```python
from build123d import *

# Parameters (mm, degrees)
BOSS_EXTRUDE1_DEPTH      = 5
BOSS_EXTRUDE1_DEPTH_BACK = 10
SKETCH1_R                = 35
M3_CLEARANCE_HOLE1_D     = 3.4
CIRPATTERN1_COUNT        = 6
SKETCH4_R                = 30
CUT_EXTRUDE1_DEPTH       = 2
M3_CLEARANCE_HOLE2_D     = 3.4
SKETCH8_R                = 35
SKETCH8_R_2              = 27.5
CUT_EXTRUDE4_DEPTH       = 4
FILLET1_R                = 0.2
SKETCH9_R                = 11.1
CUT_EXTRUDE5_DEPTH       = 10
SKETCH10_R               = 35
SKETCH10_R_2             = 27.5
CUT_EXTRUDE6_DEPTH       = 10
SKETCH11_R               = 26.5
CUT_EXTRUDE7_DEPTH       = 9
SKETCH12_R               = 11.1
CUT_EXTRUDE8_DEPTH       = 9
CHAMFER1_SIZE            = 0.2
CHAMFER2_SIZE            = 3


with BuildPart() as part:
    # Sketch1 → Boss-Extrude1 (new, two sides: drawn at the far end of the back side and taken through both)
    with BuildSketch(Plane.XY.offset(-BOSS_EXTRUDE1_DEPTH_BACK)):
        Circle(SKETCH1_R)
    extrude(amount=BOSS_EXTRUDE1_DEPTH + BOSS_EXTRUDE1_DEPTH_BACK)

    # M3 Clearance Hole1 (through all)
    with Locations(Plane.XY.offset(5)):
        with Locations((0, 32.5)):
            m3_clearance_hole1 = Hole(M3_CLEARANCE_HOLE1_D / 2)

    # CirPattern1: M3 Clearance Hole1 ×6 about axis
    cirpattern1_axis = Axis((0, -0.076854784, 0), (0, 0, 1))
    for i in range(1, CIRPATTERN1_COUNT):
        add(m3_clearance_hole1.rotate(cirpattern1_axis, i * 360 / CIRPATTERN1_COUNT), mode=Mode.SUBTRACT)

    # Sketch4 → Cut-Extrude1 (cut)
    with BuildSketch(Plane.XY.offset(5)):
        Circle(SKETCH4_R)
    extrude(amount=-CUT_EXTRUDE1_DEPTH, mode=Mode.SUBTRACT)

    # M3 Clearance Hole2 (through all)
    with Locations(Plane(origin=(-15.55, 15.55, 3), x_dir=(1, 0, 0), z_dir=(0, 0, 1))):
        with Locations((0, 0), (31.1, 0), (31.1, -31.1), (0, -31.1)):
            Hole(M3_CLEARANCE_HOLE2_D / 2)

    # Sketch8 → Cut-Extrude4 (cut)
    with BuildSketch(Plane(origin=(0, 0, -10), x_dir=(-1, 0, 0), z_dir=(0, 0, -1))):
        with Locations(Location((0, 0, 0), (0, 0, 180))):
            Circle(SKETCH8_R)
        Circle(SKETCH8_R_2, mode=Mode.SUBTRACT)
    extrude(amount=-CUT_EXTRUDE4_DEPTH, mode=Mode.SUBTRACT)

    # Fillet1
    fillet1_edges = [part.edges().sort_by_distance(p)[0] for p in [
        (-35, 0, -6),
        (27.5, 0, -10),
    ]]
    fillet(fillet1_edges, radius=FILLET1_R)

    # Sketch9 → Cut-Extrude5 (cut)
    with BuildSketch(Plane.XY.offset(3)):
        Circle(SKETCH9_R)
    extrude(amount=-CUT_EXTRUDE5_DEPTH, mode=Mode.SUBTRACT)

    # Sketch10 → Cut-Extrude6 (cut)
    with BuildSketch(Plane(origin=(0, 0, -10), x_dir=(-1, 0, 0), z_dir=(0, 0, -1))):
        with Locations(Location((0, 0, 0), (0, 0, 180))):
            Circle(SKETCH10_R)
        Circle(SKETCH10_R_2, mode=Mode.SUBTRACT)
    extrude(amount=-CUT_EXTRUDE6_DEPTH, mode=Mode.SUBTRACT)

    # Sketch11 → Cut-Extrude7 (cut)
    with BuildSketch(Plane.XY.offset(3)):
        Circle(SKETCH11_R)
    extrude(amount=-CUT_EXTRUDE7_DEPTH, mode=Mode.SUBTRACT)

    # Sketch12 → Cut-Extrude8 (cut)
    with BuildSketch(Plane.XY.offset(-7)):
        Circle(SKETCH12_R)
    extrude(amount=-CUT_EXTRUDE8_DEPTH, mode=Mode.SUBTRACT)

    # Chamfer1
    chamfer1_edges = [part.edges().sort_by_distance(p)[0] for p in [
        (-35, 0, 0),
        (-11.1, 0, -6),
    ]]
    chamfer(chamfer1_edges, length=CHAMFER1_SIZE)

    # Chamfer2
    chamfer2_edges = [part.edges().sort_by_distance(p)[0] for p in [
        (-26.5, 0, 3),
    ]]
    chamfer(chamfer2_edges, length=CHAMFER2_SIZE)


solid = part.part
```
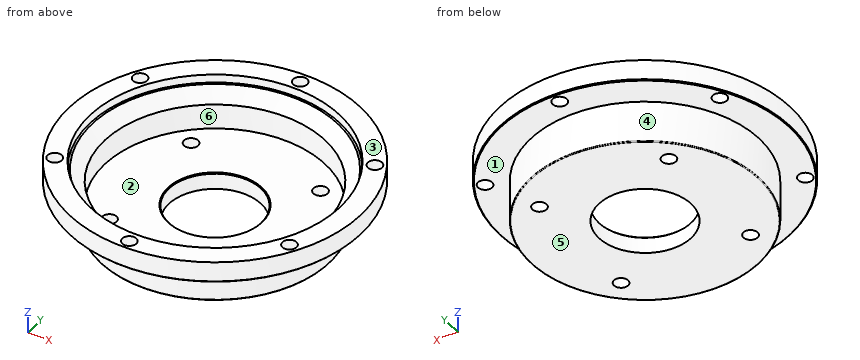
Model file for the job. Use its own axes, mm. Face numbers are marked on the shaded views. A direction names the side the tool comes from. Give positions to 0.01 mm unless a question says otherwise; leave off trailing zeros. Write each loop counter-clockwise with the first axis right and the second up, starting at its lowest first coordinate (ties: lowest second). Pieces come first, ordered by that corner, then holes. Notation, with made-up numbers: (-21, 46) - (2, 46) arc R16 cw to (2, 64) - close; hole circle Ø4 at (-18.5, -27.75). An arc over 180 degrees is marked (long way). One line per question, with ' | ' between items. Start each with the question number.
(1) Pin check, flat tips, straight feed: P1, Ø4.5, axis at x = -28.21, y = -16.37, coming from the +Z side; P2, Ø10, axis at x = 26.5, y = -21, coming from the -Z side; P3, Ø4, axis at x = -2, y = -16, coming from the +Z side; P4, Ø2, axis at x = -3, z = -2.5, coming from the +Y side. Stop position of each tip, or through.
(2) 3-axis set-ups, long thin cutter, end or side, ignore diameter. For the marked faces 1, 2 and 3: which of +Z, -Z, +X, -X, +Y, -Y reach the whole face in a straight line?
(3) Slice it at B-B on z = -8.25. Write the cut outline in (x, y), plus the area to 3 significant figures.
(4) Two-plate mould, pull along X, no slides. Class the marked faces 4, 5 and 6: +X half, -X half, draft (parallel to the pull), parting line (faces both ways), or undercut.
(5) Wall check: line 1 along Y through (x, z) = (0, 3.4); line 2 along Y through (x, z) = (0, -7.65); line 3 along Y through (x, z) = (28, 1). Give the ranges that are in metal, low to high. Write a range as from..to.
(6) Slice it at C-C on x = 15. Give the number of separate pieces and of enclosed holes in the cut face, plus the area to 3 significant figures.
(7) Slice it at A-A on y = 0. Write the cut outline in (x, z).
Results below:
1) P1: z = 5 | P2: z = 0 | P3: z = -6 | P4: y = 27.43
2) face 1: -Z | face 2: +Z | face 3: +Z, +X, -X, +Y, -Y
3) outline: circle Ø55 at (0, 0); hole circle Ø3.4 at (-15.55, -15.55); hole circle Ø3.4 at (-15.55, 15.55); hole circle Ø22.2 at (0, 0); hole circle Ø3.4 at (15.55, -15.55); hole circle Ø3.4 at (15.55, 15.55) | area: 1,950 mm^2
4) face 4: parting line | face 5: draft | face 6: undercut
5) line 1: -35..-34.35, -30.95..-30, 30..30.8, 34.2..35 | line 2: -27.5..-11.1, 11.1..27.5 | line 3: -21..-18.05, -14.68..14.52, 17.9..21
6) separate pieces: 3 | enclosed holes: 0 | area: 244 mm^2
7) outline: (-35, 0.2) - (-34.8, 0) - (-27.5, 0) - (-27.5, -9.8) arc R0.2 ccw to (-27.3, -10) - (-11.1, -10) - (-11.1, -6.2) - (-11.3, -6) - (-26.5, -6) - (-26.5, 0) - (-29.5, 3) - (-30, 3) - (-30, 5) - (-35, 5) - close; (11.1, -10) - (27.3, -10) arc R0.2 ccw to (27.5, -9.8) - (27.5, 0) - (34.8, 0) - (35, 0.2) - (35, 5) - (30, 5) - (30, 3) - (29.5, 3) - (26.5, 0) - (26.5, -6) - (11.3, -6) - (11.1, -6.2) - close
